Input: part model. Units: mm. Frame: model coordinates. A direction names the side the tool comes from. Coordinates: 2 decimals unless noted, no trailing zeros. Order: outer loops, then holes, each group sorted by start corner. A loop starts at its lowest first (then second) coordinate and runs counter-clockwise, first axis right, second up. Notation, with made-up numbers: (2, -27) -> (12, -27) arc R19 cw to (12, -12) -> close; hole circle Ø1 at (85, -34). An arc over 180 degrees is marked (long way). One line per question, with ' | ' between items.
```python
from build123d import *

# Parameters (mm, degrees)
SKETCH1_W           = 7.11
SKETCH1_H           = 3.68
BOSS_EXTRUDE1_DEPTH = 7.01
SKETCH2_R           = 1.75
BOSS_EXTRUDE2_DEPTH = 5.74
SKETCH3_R           = 0.45
BOSS_EXTRUDE3_DEPTH = 1.5


with BuildPart() as part:
    # Sketch1 → Boss-Extrude1 (new body)
    with BuildSketch(Plane(origin=(0, 0, 0), x_dir=(1, 0, 0), z_dir=(0, 1, 0))):
        Rectangle(SKETCH1_W, SKETCH1_H)
    extrude(amount=BOSS_EXTRUDE1_DEPTH)

    # Sketch2 → Boss-Extrude2 (add)
    with BuildSketch(Plane.XY.offset(1.84)):
        with Locations(Location((0, 4, 0), (0, 0, 180))):
            Circle(SKETCH2_R)
    extrude(amount=BOSS_EXTRUDE2_DEPTH)

    # Sketch3 → Boss-Extrude3 (add)
    with BuildSketch(Plane(origin=(0, 0, 0), x_dir=(1, 0, 0), z_dir=(0, 1, 0))):
        with Locations(Location((-2.245, 0.77, 0), (0, 0, 270))):
            Circle(SKETCH3_R)
        with Locations(Location((2.245, 0.77, 0), (0, 0, 270))):
            Circle(SKETCH3_R)
    extrude(amount=-BOSS_EXTRUDE3_DEPTH)


solid = part.part
```
1. Access query for faces 4 (the face through (0.38, 5.71, 4.67)), 5 (the face through (-1.94, -0.74, -1.1)), 6 (the face through (0, 3, -1.84)). Directions: +Z, -Z, +X, -X, +Y, -Y. A direction counts if a zero-diameter tool reaches every point of the face in a straight line with its end or side. Return the directions, or none.
Recorded:
face 4: +Z | face 5: -Y | face 6: -Z, +X, -X, +Y, -Y
2. Pin query (flat end, axial travel): pin 1 Ø1 at (y, z) = (4.5, 3.5) entering from -X; pin 2 Ø2 at (x, z) = (2.5, 3) entering from -Y; pin 3 Ø1.5 at (x, z) = (2, 3.5) entering from -Y. Return the tip coordinate at first contact, or that it passes through.
Recorded:
pin 1: stops at x = -1.75 | pin 2: stops at y = 3.1 | pin 3: stops at y = 2.78
3. Cut plane B-B, the plane x = 0. Return loops of the section in (y, z).
Recorded:
outline: (0, -1.84) -> (7.01, -1.84) -> (7.01, 1.84) -> (5.75, 1.84) -> (5.75, 7.58) -> (2.25, 7.58) -> (2.25, 1.84) -> (0, 1.84) -> close
4. Cut plane A-A, the plane z = -0.77. Return loops of the section in (x, y) (3 decimals).
Recorded:
outline: (-3.555, 0) -> (-2.695, 0) -> (-2.695, -1.5) -> (-1.795, -1.5) -> (-1.795, 0) -> (1.795, 0) -> (1.795, -1.5) -> (2.695, -1.5) -> (2.695, 0) -> (3.555, 0) -> (3.555, 7.01) -> (-3.555, 7.01) -> close
5. Mould query, pull axis X, two halves, no side actions, for faces 1 (the face through (0, 0, 0)), 2 (the face through (0, 2, 1.84)), 3 (the face through (-3.555, 3, 0)). Classes: released by +X, released by -X, zero draft, split by the parting line, or undercut.
Recorded:
face 1: undercut | face 2: zero draft | face 3: released by -X
6. Cut plane C-C, the plane y = 5.5. Return loops of the section in (x, z) (3 decimals).
Recorded:
outline: (-3.555, -1.84) -> (3.555, -1.84) -> (3.555, 1.84) -> (0.901, 1.84) -> (0.901, 7.58) -> (-0.901, 7.58) -> (-0.901, 1.84) -> (-3.555, 1.84) -> close
7. Cut plane D-D, the plane z = 0.75. Return loops of the section in (x, y) (3 decimals).
Recorded:
outline: (-3.555, 0) -> (3.555, 0) -> (3.555, 7.01) -> (-3.555, 7.01) -> close
8. Ray query, line 1 (X direction, y = -1, z = -0.75); line 2 (Z direction, x = -3, y = 4); line 3 (Y direction, x = -3, z = -1). Return the intervals inside material, ascending. Write a range as [from, to].
Recorded:
line 1: x = [-2.69, -1.8], [1.8, 2.69] | line 2: z = [-1.84, 1.84] | line 3: y = [0, 7.01]
